Autodesk Inventor part; units mm, degrees
ref_plane "YZ Plane" through (0, 0, 0) normal (1, 0, 0) x (0, 1, 0)
ref_plane "XZ Plane" through (0, 0, 0) normal (0, 1, 0) x (-1, 0, 0)
ref_plane "XY Plane" through (0, 0, 0) normal (0, 0, 1) x (1, 0, 0)
sketch "Sketch1" plane through (0, 0, 0) normal (0, 1, 0) x (-1, 0, 0)
  line L0 (-10, -60) -> (-105, -60)
  line L1 (-115, -50) -> (-115, -10)
  line L2 (-105, 0) -> (-10, 0)
  line L3 (0, -10) -> (0, -50)
  arc A0 (-10, -60) -> (0, -50) centre (-10, -50) ccw
  arc A1 (0, -10) -> (-10, 0) centre (-10, -10) ccw
  arc A2 (-115, -50) -> (-105, -60) centre (-105, -50) ccw
  arc A3 (-105, 0) -> (-115, -10) centre (-105, -10) ccw
  point P0 (0, 0)
  point P1 (0, -60)
  point P2 (-115, 0)
  point P3 (-115, -60)
  point P4 (0, 0)
  dimension "d0" = 115
  dimension "d1" = 60
  dimension "d29" = 10
extrude "Extrusion1" add sketch "Sketch1" along normal blind 4
sketch "Sketch2" plane through (0, 4, 0) normal (0, 1, 0) x (1, 0, 0)
  circle A0 centre (20, 55) radius 1.75
  line L0 (105, 60) -> (10, 60)
  line L1 (0, 50) -> (0, 0)
  circle A1 centre (105, 55) radius 1.75
  circle A2 centre (20, 5) radius 1.75
  circle A3 centre (105, 5) radius 1.75
  circle A4 centre (102.5, 42.5) radius 1.75
  circle A5 centre (102.5, 17.5) radius 1.75
  line L2 (115, 10) -> (115, 50)
  circle A6 centre (64.5, 47) radius 1.75
  circle A7 centre (64.5, 13) radius 1.75
  point P0 (115, 60)
  point P1 (0, 60)
  point P2 (115, 0)
  dimension "d4" = 3.5
  dimension "d5" = 5
  dimension "d6" = 20
  dimension "d9" = 85
  dimension "d12" = 50
  dimension "d15" = 3.5
  dimension "d16" = 3.5
  dimension "d17" = 25
  dimension "d18" = 0
  dimension "d19" = 12.5
  dimension "d20" = 3.5
  dimension "d21" = 3.5
  dimension "d22" = 34
  dimension "d23" = 0
  dimension "d24" = 38
  dimension "d25" = 17.5
  dimension "d26" = 13
extrude "Extrusion2" cut sketch "Sketch2" against normal through all
properties part number "rfid_cover"
The listing builds one solid part. Answer for the finished solid, in the listing's coordinates (mm). Coordinates: 2 decimals unless noted, no trailing zeros. Order: outer loops, then holes, each group sorted by start corner. A loop starts at its lowest first (then second) coordinate and runs counter-clockwise, first axis right, second up. Notation, with made-up numbers: (78.25, -14.75) -> (102.25, -14.75) arc R25 ccw to (102.25, -1.75) -> close; hole circle Ø4 at (71.5, -3.75). An arc over 180 degrees is marked (long way). Answer in a Markdown table with one row per item. Add a question column.
Item 1: Determine the mould class of faces 1 (the face through (18.61, 2.03, -3.94)), 2 (the face through (2.85, 1.97, -56.99)), 3 (the face through (57, 2, -60)), 4 (the face through (111.99, 1.97, -57.15)) for opening direction X: +X half, -X half, draft (parallel to the pull), parting line (faces both ways), or undercut.
Item 2: Find section C-C (y = 3.25). State how many separate pieces and enclosed holes the cut face has, then the cut area to 3 significant figures.
Item 3: This flat-tipped pin is pushed along its axis until it touches: P1, Ø3, axis at x = 102.5, z = -17.5, coming from the -Y side. Where does it stop, or does it pass through?
Item 4: Find the intervals of material crossed by L1, parallel to Z at x = 20, y = 2.2; L2, parallel to Z at x = 102.5, y = 2.55; L3, parallel to X at y = 2.2, z = -47, in increasing order. Write a range as from..to.
Item 5: Find section D-D (z = -55). Write down the section's boundary in (x, y), then the cut area to 3 significant figures.
Item 6: Find section A-A (x = 20). Write down the section's boundary in (y, z).
Item 7: Find section B-B (z = -42.5). Write down the section's boundary in (x, y).
Result set:
| question | item | result |
|---|---|---|
| 1 | face 1 | undercut |
| 1 | face 2 | -X half |
| 1 | face 3 | draft |
| 1 | face 4 | +X half |
| 2 | separate pieces | 1 |
| 2 | enclosed holes | 8 |
| 2 | area | 6,740 mm² |
| 3 | P1 | passes through |
| 4 | L1 | z = -60..-56.75, -53.25..-6.75, -3.25..0 |
| 4 | L2 | z = -60..-44.25, -40.75..-19.25, -15.75..0 |
| 4 | L3 | x = 0..62.75, 66.25..115 |
| 5 | outline | (1.34, 0) -> (18.25, 0) -> (18.25, 4) -> (1.34, 4) -> close; (21.75, 0) -> (103.25, 0) -> (103.25, 4) -> (21.75, 4) -> close; (106.75, 0) -> (113.66, 0) -> (113.66, 4) -> (106.75, 4) -> close |
| 5 | area | 421 mm² |
| 6 | outline | (0, -60) -> (4, -60) -> (4, -56.75) -> (0, -56.75) -> close; (0, -53.25) -> (4, -53.25) -> (4, -6.75) -> (0, -6.75) -> close; (0, -3.25) -> (4, -3.25) -> (4, 0) -> (0, 0) -> close |
| 7 | outline | (0, 0) -> (100.75, 0) -> (100.75, 4) -> (0, 4) -> close; (104.25, 0) -> (115, 0) -> (115, 4) -> (104.25, 4) -> close |
